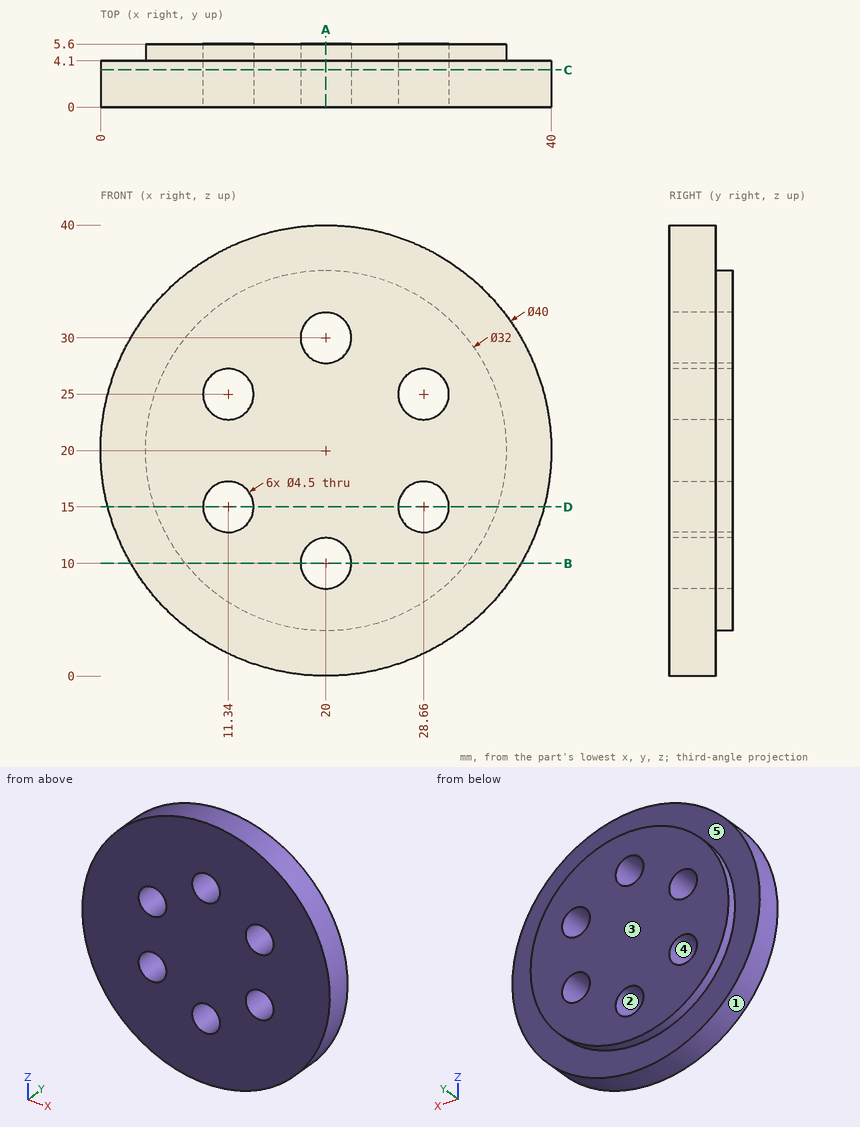
Drawing for the job (mm, zero at the part's lowest x, y, z). A direction names the side the tool comes from. Round coordinates to 2 decimals unless told otherwise and drop trailing zeros. Write each loop counter-clockwise with the first axis right and the second up, starting at its lowest first coordinate (ties: lowest second). Pieces come first, ordered by that corner, then holes. Notation, with made-up numbers: M 46.25,11.5 L 77.25,11.5 A10 cw 77.25,20.5 Z; hole C 3,27 d8. An arc over 180 degrees is marked long. Answer as a JSON object with one key per item and string values. Group by question number.
(1) Cut at A-A (x = 20). Give the cut face in (y, z), and give its area (3 significant figures).
(2) Mould opens along X. For the marked faces 1, 2 and 3 say: pulls with the +X half, pulls with the -X half, needs draft (parallel to the pull), parting line crosses it, or undercut.
(3) Which spindle directions (+Z, -Z, +X, -X, +Y, -Y) get a long thin tool onto all of the face, cutting with end or side? Do the marked faces 4 and 5. Say none if no direction does.
(4) Drill centre lines: L1, parallel to X at y = 3.4, z = 25 (1 decimal); L2, parallel to Z at x = 21, y = 2.65 (1 decimal); L3, parallel to Z at x = 29, y = 4.85 (1 decimal). Where is each one in solid material? Low to high.
(5) Cut at D-D (z = 15). Give the cut face in (x, y) (1 decimal), and give its area (3 significant figures).
(6) Cut at C-C (y = 3.3). Give the cut face in (x, z), and give its area (3 significant figures).
(7) Flat gauge pins, fed straight in: pin 1 (1.5 mm diameter, centred on x = 4.5, z = 13, fed in from +Y); pin 2 (2 mm diameter, centred on y = 1, z = 27.5, fed in from -X); pin 3 (1.5 mm diameter, centred on y = 2, z = 26.5, fed in from +X). Where does each tip first touch, or does it go through?
(8) Cut at B-B (z = 10). Give the cut face in (x, y).
Responses:
{
 "1": {"outline": "M 0,0 L 4.1,0 L 4.1,4 L 5.6,4 L 5.6,7.75 L 0,7.75 Z; M 0,12.25 L 5.6,12.25 L 5.6,27.75 L 0,27.75 Z; M 0,32.25 L 5.6,32.25 L 5.6,36 L 4.1,36 L 4.1,40 L 0,40 Z", "area": "162 mm2"},
 "2": {"face 1": "parting line crosses it", "face 2": "undercut", "face 3": "needs draft"},
 "3": {"face 4": "+Y, -Y", "face 5": "+Y"},
 "4": {"L1": "x = 0.6 to 9.1, 13.6 to 26.4, 30.9 to 39.4", "L2": "z = 0 to 8, 12 to 28, 32 to 40", "L3": "z = 6.8 to 12.8, 17.2 to 22.8, 27.2 to 33.2"},
 "5": {"outline": "M 0.6,0 L 9.1,0 L 9.1,5.6 L 4.8,5.6 L 4.8,4.1 L 0.6,4.1 Z; M 13.6,0 L 26.4,0 L 26.4,5.6 L 13.6,5.6 Z; M 30.9,0 L 39.4,0 L 39.4,4.1 L 35.2,4.1 L 35.2,5.6 L 30.9,5.6 Z", "area": "154 mm2"},
 "6": {"outline": "C 20,20 d40; hole C 11.34,15 d4.5; hole C 11.34,25 d4.5; hole C 20,10 d4.5; hole C 20,30 d4.5; hole C 28.66,15 d4.5; hole C 28.66,25 d4.5", "area": "1,160 mm2"},
 "7": {"pin 1": "stops at y = 4.1", "pin 2": "stops at x = 1.09", "pin 3": "stops at x = 39.16"},
 "8": {"outline": "M 2.68,0 L 17.75,0 L 17.75,5.6 L 7.51,5.6 L 7.51,4.1 L 2.68,4.1 Z; M 22.25,0 L 37.32,0 L 37.32,4.1 L 32.49,4.1 L 32.49,5.6 L 22.25,5.6 Z"}
}
